Model file for the job. Use its own axes, mm. A direction names the side the tool comes from. Give positions to 0.01 mm unless a question says otherwise; leave off trailing zeros. Order: outer loops, then holes, each group sorted by start corner. A loop starts at its lowest first (then second) coordinate and runs counter-clockwise, first axis right, second up. Notation, with made-up numbers: (23, 37) -> (70, 37) arc R23 ccw to (70, 69) -> close; hole circle Ø10 at (88.25, 39.5). An arc over 180 degrees is marked (long way). Use CSV: the item, a comma, the result in double quotes. Start each with the question number.
1. Cut at A-A on x = 0. List the corners of the cut face in (y, z).
2. Drop flat-ended pins along their axis: pin 1 (5 mm diameter, centred on x = 18.5, z = -7.5, fed in from -Y); pin 2 (2 mm diameter, centred on y = -9, z = 14, fed in from -X); pin 3 (17 mm diameter, centred on x = 0, y = 0, fed in from +Z). Give the stop position or say it passes through.
3. Wall check: line 1 (Y direction, x = -12.5, z = -6.5); line 2 (X direction, y = 35, z = -6); line 3 (Z direction, x = 47.5, y = -6.5). Give the ranges that are in metal, low to high. Write a range as from..to.
4. Cut at C-C on z = 5. List the corners of the cut face in (x, y), then the cut area to 3 significant figures.
5. 3-axis set-ups, long thin cutter, end or side, ignore diameter. For faces 1 (the flat face through (-11, -1, 15)), 2 (the flat face through (-36, 41, 20.5)), 3 (the cylindrical face through (-11.706, 52.716, -17.712)), 4 (the flat face through (-25, 10, 0)): which of +Z, -Z, +X, -X, +Y, -Y reach the whole face in a straight line?
6. Cut at D-D on y = -30. Give the number of separate pieces and of enclosed holes in the cut face, then the cut area to 3 significant figures.
```python
from build123d import *

# Parameters (mm, degrees)
SKETCH3_W               = 80
SKETCH3_H               = 30
BOSS_EXTRUDE3_DEPTH     = 10
SKETCH5_W               = 30
SKETCH5_H               = 80
BOSS_EXTRUDE4_DEPTH     = 10
CUT_EXTRUDE1_DEPTH      = 115.990220301
CUT_EXTRUDE1_DEPTH_BACK = 115.990220301
SKETCH7_R               = 7.5


with BuildPart() as part:
    # Sketch1 → Revolve1 (revolve)
    with BuildSketch(Plane(origin=(0, 0, 0), x_dir=(1, 0, 0), z_dir=(0, 1, 0))):
        with BuildLine():
            Line((40, 15), (40, -15))
            Line((40, -15), (54, -15))
            Line((54, -15), (54, -20.5))
            Line((54, -20.5), (70, -20.5))
            ThreePointArc((70, -20.5), (80.007814408, 0), (70, 20.5))
            Line((70, 20.5), (54, 20.5))
            Line((54, 20.5), (54, 15))
            Line((54, 15), (40, 15))
        make_face()
    revolve(axis=Axis((0, 0, 7131.725244947), (0, 0, -1)))

    # Sketch3 → Boss-Extrude3 (add, symmetric)
    with BuildSketch(Plane(origin=(0, 0, 0), x_dir=(1, 0, 0), z_dir=(0, 1, 0))):
        Rectangle(SKETCH3_W, SKETCH3_H)
    extrude(amount=BOSS_EXTRUDE3_DEPTH, both=True)

    # Sketch5 → Boss-Extrude4 (add, symmetric)
    with BuildSketch(Plane(origin=(0, 0, 0), x_dir=(0, 0, -1), z_dir=(1, 0, 0))):
        Rectangle(SKETCH5_W, SKETCH5_H)
    extrude(amount=BOSS_EXTRUDE4_DEPTH, both=True)

    # Sketch7 → Cut-Extrude1 (cut, two sides: drawn at the far end of the back side and taken through both)
    with BuildSketch(Plane.XY.offset(-CUT_EXTRUDE1_DEPTH_BACK)):
        Circle(SKETCH7_R)
    extrude(amount=CUT_EXTRUDE1_DEPTH + CUT_EXTRUDE1_DEPTH_BACK, mode=Mode.SUBTRACT)


solid = part.part
```
Verdict:
1,outline,"(-70, -20.5) -> (-54, -20.5) -> (-54, -15) -> (-7.5, -15) -> (-7.5, 15) -> (-54, 15) -> (-54, 20.5) -> (-70, 20.5) arc R26 ccw to start; (7.5, -15) -> (54, -15) -> (54, -20.5) -> (70, -20.5) arc R26 ccw to (70, 20.5) -> (54, 20.5) -> (54, 15) -> (7.5, 15) -> close"
2,pin 1,"y = -77.58"
2,pin 2,"x = -76.01"
2,pin 3,"z = 15"
3,line 1,"-78.19..-38, -10..10, 38..78.19"
3,line 2,"-71.16..-19.36, -10..10, 19.36..71.16"
3,line 3,"-15..15"
4,outline,"circle Ø159.05 at (0, 0); hole (-38.73, -10) arc R40 ccw to (-10, -38.73) -> (-10, -10) -> close; hole (-38.73, 10) -> (-10, 10) -> (-10, 38.73) arc R40 ccw to start; hole circle Ø15 at (0, 0); hole (10, -38.73) arc R40 ccw to (38.73, -10) -> (10, -10) -> close; hole (10, 10) -> (38.73, 10) arc R40 ccw to (10, 38.73) -> close"
4,area,"17,400 mm^2"
5,face 1,"+Z"
5,face 2,"+Z, +X, -X, +Y, -Y"
5,face 3,"-Z"
5,face 4,"+Z, -Z"
6,separate pieces,"3"
6,enclosed holes,"0"
6,area,"3,840 mm^2"
